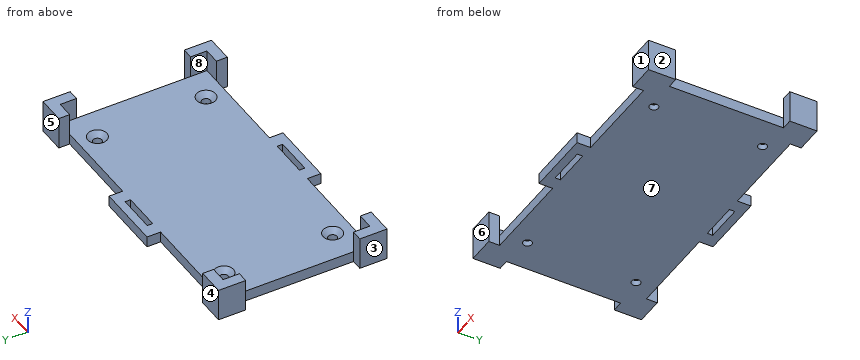
```python
from build123d import *

# Parameters (mm, degrees)
SKETCH_W                = 103
SKETCH_H                = 54
PAD_DEPTH               = 4
PAD001_DEPTH            = 12
PAD001_MIRRORED_2_DEPTH = 12
POLARPATTERN_COUNT      = 2
HOLE_D                  = 3.2
HOLE_CSINK_D            = 7
HOLE_CSINK_ANGLE        = 90
PAD002_DEPTH            = 4


with BuildPart() as part:
    # Sketch → Pad (new body)
    with BuildSketch(Plane.XY):
        Rectangle(SKETCH_W, SKETCH_H)
    extrude(amount=PAD_DEPTH)

    # Sketch001 → Pad001 (join)
    with BuildSketch(Plane.XY):
        Polygon((-51.5, 21), (-51.5, 27), (-45.5, 27), (-45.5, 31), (-55.5, 31), (-55.5, 21), align=None)
    pad001 = extrude(amount=PAD001_DEPTH)

    # Sketch001 Mirrored 2 → Pad001 Mirrored 2 (add)
    with BuildSketch(Plane(origin=(0, 0, 0), x_dir=(-1, 0, 0), z_dir=(0, 0, -1))):
        Polygon((-51.5, 21), (-51.5, 27), (-45.5, 27), (-45.5, 31), (-55.5, 31), (-55.5, 21), align=None)
    pad001_mirrored_2 = extrude(amount=-PAD001_MIRRORED_2_DEPTH)

    # PolarPattern: Pad001, Pad001 Mirrored 2 ×2 about axis
    polarpattern_axis = Axis((0, 0, 0), (0, 0, 1))
    for i in range(1, POLARPATTERN_COUNT):
        add(pad001.rotate(polarpattern_axis, i * 360 / POLARPATTERN_COUNT))
        add(pad001_mirrored_2.rotate(polarpattern_axis, i * 360 / POLARPATTERN_COUNT))

    # Hole (through all)
    with Locations(Plane.XY.offset(4)):
        with Locations((-40, 20), (40, 20), (40, -20), (-40, -20)):
            CounterSinkHole(HOLE_D / 2, HOLE_CSINK_D / 2, counter_sink_angle=HOLE_CSINK_ANGLE)

    # Sketch004 → Pad002 (join)
    with BuildSketch(Plane.XY):
        Polygon((-7, 27), (-7, 29), (7, 29), (7, 27), (12, 27), (12, 32), (-12, 32), (-12, 27), align=None)
    pad002 = extrude(amount=PAD002_DEPTH)

    # Mirrored001: Pad002 across XZ
    add(pad002.mirror(Plane.XZ))


solid = part.part
```
Model file for the job. Use its own axes, mm. Face numbers are marked on the shaded views. A direction names the side the tool comes from. Coordinates: 2 decimals unless noted, no trailing zeros. Write each loop counter-clockwise with the first axis right and the second up, starting at its lowest first coordinate (ties: lowest second). Pieces come first, ordered by that corner, then holes. Notation, with made-up numbers: (45.5, 38.25) - (101.5, 38.25) arc R22 cw to (101.5, 54.25) - close; hole circle Ø6 at (79, 16.5). An arc over 180 degrees is marked (long way). One line per item, written item: value. Start each with the question number.
1. Slice it at A-A (x = 3.5). Write the cut outline in (y, z), plus the area to 3 significant figures.
2. Probe line 1 (Y direction, x = -40, z = 1.55); line 2 (Y direction, x = 5.5, z = 3.5); line 3 (X direction, y = -20, z = 1.05). List the from-to ranges inside material, lowest first. Write a range as from..to.
3. Flat gauge pins, fed straight in: pin 1 (3 mm diameter, centred on x = 1.5, z = 6.5, fed in from -Y); pin 2 (3 mm diameter, centred on x = 48, z = 6, fed in from -Y); pin 3 (10 mm diameter, centred on x = 11.5, y = -19.5, fed in from +Z); pin 4 (5 mm diameter, centred on x = -40, y = -20, fed in from +Z). Where does each tip first touch, or does it go through?
4. Mould opens along Y. For the marked faces 6, 7 and 8 say: released by +Y, released by -Y, zero draft, split by the parting line, or undercut.
5. Slice it at D-D (y = 6.5). Write the cut outline in (x, z).
6. Slice it at B-B (z = 9). Write the cut outline in (x, y), plus the area to 3 significant figures.
7. Slice it at C-C (x = -40). Write the cut outline in (y, z).
8. Tool access for the marked faces 1, 2, 3, 4 and 5: list every direction of +Z, -Z, +X, -X, +Y, -Y with a clear straight run to the whole face (end or side of a thin tool).
Answers below:
1. outline: (-32, 0) - (-29, 0) - (-29, 4) - (-32, 4) - close; (-27, 0) - (27, 0) - (27, 4) - (-27, 4) - close; (29, 0) - (32, 0) - (32, 4) - (29, 4) - close
1. area: 240 mm^2
2. line 1: y = -27..-21.6, -18.4..18.4, 21.6..27
2. line 2: y = -32..-29, -27..27, 29..32
2. line 3: x = -51.5..-41.6, -38.4..38.4, 41.6..51.5
3. pin 1: passes through
3. pin 2: stops at y = -31
3. pin 3: stops at z = 4
3. pin 4: stops at z = 3
4. face 6: released by -Y
4. face 7: zero draft
4. face 8: undercut
5. outline: (-51.5, 0) - (51.5, 0) - (51.5, 4) - (-51.5, 4) - close
6. outline: (-55.5, -31) - (-45.5, -31) - (-45.5, -27) - (-51.5, -27) - (-51.5, -21) - (-55.5, -21) - close; (-55.5, 21) - (-51.5, 21) - (-51.5, 27) - (-45.5, 27) - (-45.5, 31) - (-55.5, 31) - close; (45.5, -31) - (55.5, -31) - (55.5, -21) - (51.5, -21) - (51.5, -27) - (45.5, -27) - close; (45.5, 27) - (51.5, 27) - (51.5, 21) - (55.5, 21) - (55.5, 31) - (45.5, 31) - close
6. area: 256 mm^2
7. outline: (-27, 0) - (-21.6, 0) - (-21.6, 2.1) - (-23.5, 4) - (-27, 4) - close; (-18.4, 0) - (18.4, 0) - (18.4, 2.1) - (16.5, 4) - (-16.5, 4) - (-18.4, 2.1) - close; (21.6, 0) - (27, 0) - (27, 4) - (23.5, 4) - (21.6, 2.1) - close
8. face 1: +Z, -Z, +X, -Y
8. face 2: +Z, -Z, +X, +Y, -Y
8. face 3: +Z, -Z, -X, +Y, -Y
8. face 4: +Z, -Z, -X, +Y
8. face 5: +Z, -Z, +X, +Y
